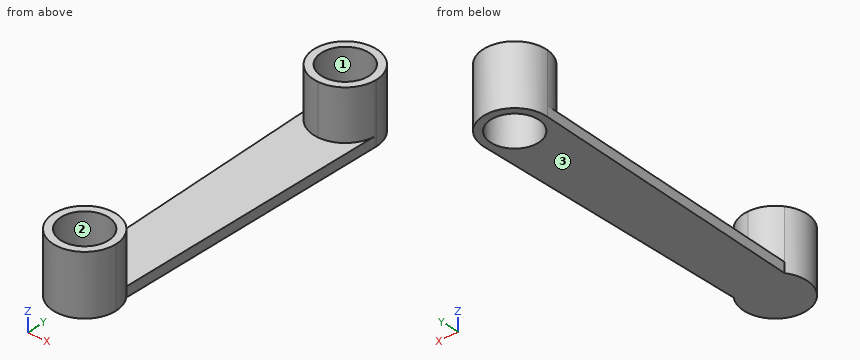
```python
from build123d import *

# Parameters (mm, degrees)
F1_DEPTH = 2
F0_R     = 4.75
F2_DEPTH = 12


with BuildPart() as f1:
    # F0 (on Top) → F1 (new body)
    with BuildSketch(Plane.XY):
        with BuildLine():
            Line((-6.2413531605, 22.5833728044), (-5.0444387575, -32.6162494679))
            ThreePointArc((-5.0444387575, -32.6162494679), (-2.8284243086, -30.7328789341), (0, -30.0562545657))
            Line((0, -30.0562545657), (0, 16.6620226577))
            ThreePointArc((0, 16.6620226577), (-4.3016530786, 18.3778986197), (-6.2413531605, 22.5833728044))
        make_face()
        with BuildLine():
            ThreePointArc((0, -30.0562545657), (2.8284243086, -30.7328789341), (5.0444387575, -32.6162494679))
            Line((5.0444387575, -32.6162494679), (6.2413531605, 22.5833728044))
            ThreePointArc((6.2413531605, 22.5833728044), (4.3016530786, 18.3778986197), (0, 16.6620226577))
            Line((0, 16.6620226577), (0, -30.0562545657))
        make_face()
    extrude(amount=F1_DEPTH)



with BuildPart() as f1b:
    # F0 (on Top) → F1, piece 2 (new body)
    with BuildSketch(Plane.XY):
        with Locations((0, -36.3062545657)):
            Circle(F0_R)
    extrude(amount=F1_DEPTH)


with BuildPart() as f1_1:
    add(f1.part)

    add(f1b.part)  # F2 merges F1b
    # F0 (on Top) → F2 (join)
    with BuildSketch(Plane.XY):
        with BuildLine():
            ThreePointArc((0, 16.6620226577), (4.3016530786, 18.3778986197), (6.2413531605, 22.5833728044))
            ThreePointArc((6.2413531605, 22.5833728044), (6.2478379162, 22.7476408659), (6.25, 22.9120226577))
            ThreePointArc((6.25, 22.9120226577), (-0.1643817918, 29.1598605738), (-6.2413531605, 22.5833728044))
            ThreePointArc((-6.2413531605, 22.5833728044), (-4.3016530786, 18.3778986197), (0, 16.6620226577))
        make_face()
        with Locations((0, 22.9120226577)):
            Circle(F0_R, mode=Mode.SUBTRACT)
        with BuildLine():
            ThreePointArc((-5.0444387575, -32.6162494679), (-1.9409736945, -42.2472242776), (6.25, -36.3062545657))
            ThreePointArc((6.25, -36.3062545657), (5.9409697119, -34.3652808712), (5.0444387575, -32.6162494679))
            ThreePointArc((5.0444387575, -32.6162494679), (2.8284243086, -30.7328789341), (0, -30.0562545657))
            ThreePointArc((0, -30.0562545657), (-2.8284243086, -30.7328789341), (-5.0444387575, -32.6162494679))
        make_face()
        with Locations((0, -36.3062545657)):
            Circle(F0_R, mode=Mode.SUBTRACT)
    extrude(amount=F2_DEPTH)


solid = f1_1.part
```
Read the model definition and answer for the solid it produces. Units are mm, in the model's axes. Face numbers are marked on the shaded views. Coordinates: 2 decimals unless noted, no trailing zeros. Write each loop counter-clockwise with the first axis right and the second up, starting at its lowest first coordinate (ties: lowest second). Pieces come first, ordered by that corner, then holes. Notation, with made-up numbers: (-32.5, -31.5) -> (23.5, -31.5) arc R17 ccw to (23.5, -6.5) -> close; hole circle Ø6 at (3, -37). An arc over 180 degrees is marked (long way). Answer as a JSON object with one key per item and string values.
Q1. The part is cut by section D-D on y = -17.5. Give the vertices of the cut face in (x, z).
The answers:
{"outline": "(-5.37, 0) -> (5.37, 0) -> (5.37, 2) -> (-5.37, 2) -> close"}
Q2. Flat-ended cylindrical pins translate along their axes: pin 1 Ø2 at (x, z) = (-4.5, 6) entering from -Y; pin 2 Ø6 at (x, y) = (2.5, -17.5) entering from +Z; pin 3 Ø2 at (x, z) = (4.5, 9) entering from +Y. Find the tip coordinate at first contact, or state that the pin passes through.
The answers:
{"pin 1": "stops at y = -41.48", "pin 2": "stops at z = 2", "pin 3": "stops at y = 28.09"}
Q3. Consider line 1 (Y direction, x = 0, z = 7); line 2 (Y direction, x = -0.25, z = 5.25); line 3 (Y direction, x = 3, z = 0.75). Determine where each line is inside the solid, lowest interval first. Write a range as [from, to].
The answers:
{"line 1": "y = [-42.56, -41.06], [-31.56, -30.06], [16.66, 18.16], [27.66, 29.16]", "line 2": "y = [-42.55, -41.05], [-31.56, -30.06], [16.67, 18.17], [27.66, 29.16]", "line 3": "y = [-41.79, 19.23], [26.59, 28.39]"}
Q4. The part is cut by section C-C on x = 2.5. Give the vertices of the cut face in (y, z), then the cut area to 3 significant figures.
The answers:
{"outline": "(-42.03, 0) -> (18.87, 0) -> (18.87, 12) -> (17.18, 12) -> (17.18, 2) -> (-30.58, 2) -> (-30.58, 12) -> (-32.27, 12) -> (-32.27, 2) -> (-40.35, 2) -> (-40.35, 12) -> (-42.03, 12) -> close; (26.95, 0) -> (28.64, 0) -> (28.64, 12) -> (26.95, 12) -> close", "area": "193 mm2"}
Q5. The part is cut by section B-B on y = 19.5. Give the vertices of the cut face in (x, z), then the cut area to 3 significant figures.
The answers:
{"outline": "(-6.17, 0) -> (-3.3, 0) -> (-3.3, 12) -> (-5.24, 12) -> (-5.24, 2) -> (-6.17, 2) -> close; (3.3, 0) -> (6.17, 0) -> (6.17, 2) -> (5.24, 2) -> (5.24, 12) -> (3.3, 12) -> close", "area": "50.1 mm2"}
Q6. Determine the mould class of the marked faces 1, 2 and 3 for opening direction Y: pulls with the +Y half, pulls with the -Y half, needs draft (parallel to the pull), parting line crosses it, or undercut.
The answers:
{"face 1": "undercut", "face 2": "undercut", "face 3": "needs draft"}
Q7. The part is cut by section A-A on z = 6. Give the vertices of the cut face in (x, y).
The answers:
{"outline": "circle Ø12.5 at (0, -36.31); circle Ø12.5 at (0, 22.91); hole circle Ø9.5 at (0, -36.31); hole circle Ø9.5 at (0, 22.91)"}
